Build history of the part. All positions in model axes, mm. A direction names the side the tool comes from. Coordinates: 2 decimals unless noted, no trailing zeros. Order: outer loops, then holes, each group sorted by start corner. A loop starts at its lowest first (then second) coordinate and runs counter-clockwise, first axis right, second up. Notation, with made-up numbers: M 41,-20 L 68,-20 A28 ccw 68,16 Z; hole C 10.5,-1 d6. An arc over 180 degrees is marked long. Write item = value, one per line. Start each with the question number.
Q1. Drill centre lines: probe 1 along X at (y, z) = (0.95, 6.17); probe 2 along Z at (x, y) = (5, 0.1); probe 3 along Z at (x, y) = (4.5, 0.5). Where is each one in solid material? Low to high.
Q2. Band-saw the part on D-D on x = 6.5. Write the cut outline in (y, z).
Q3. Band-saw the part on B-B on z = 4. Write the cut outline in (x, y), plus the area to 3 significant figures.
Q4. 3-axis set-ups, long thin cutter, end or side, ignore diameter. For faces 5 (the face through (15.51, 1.08, 3.37)), 6 (the face through (4, 1, 12.65)): which of +Z, -Z, +X, -X, +Y, -Y reach the whole face in a straight line?
Q5. Pull direction Z, two halves, no side cores. Call faces 1 (the face through (3.51, 1.08, 3.37)), 2 (the face through (20, 1, 17)), 3 (the face through (9.85, 1.08, 27)), 4 (the face through (10, 1, 0)): released by +Z, released by -Z, zero draft, split by the parting line, or undercut.
Q6. Band-saw the part on C-C on y = 1.65. Write the cut outline in (x, z).
Q7. Pin check, flat tip, straight feed: P1, Ø1.4, axis at x = 4, z = 4, coming from the -Y side. Stop position of the tip, or through.
Q8. Band-saw the part on A-A on x = 4. Write the cut outline in (y, z).
```python
from build123d import *

# Parameters (mm, degrees)
SKETCH_1_R      = 0.8
SKETCH_1_R_2    = 0.4
EXTRUDE_1_DEPTH = 2.2


with BuildPart() as part:
    # 草图1 → 凸台-拉伸1 (new body)
    with BuildSketch(Plane(origin=(0, 0, 0), x_dir=(1, 0, 0), z_dir=(0, 1, 0))):
        with BuildLine():
            Line((20, 0), (0, 0))
            Line((0, 0), (0, -12.65))
            Line((0, -12.65), (8.608058909, -12.65))
            ThreePointArc((8.608058909, -12.65), (12.283882181, -13.116117819), (14, -16.4))
            ThreePointArc((14, -16.4), (12.283882181, -19.683882181), (8.608058909, -20.15))
            Line((8.608058909, -20.15), (0, -20.15))
            Line((0, -20.15), (0, -32.8))
            Line((0, -32.8), (20, -32.8))
            Line((20, -32.8), (20, 0))
        make_face()
        with Locations(Location((4, -28.8, 0), (0, 0, 270))):
            Circle(SKETCH_1_R, mode=Mode.SUBTRACT)
        with Locations(Location((10, -26.63, 0), (0, 0, 270))):
            Circle(SKETCH_1_R_2, mode=Mode.SUBTRACT)
        with Locations(Location((16, -28.8, 0), (0, 0, 270))):
            Circle(SKETCH_1_R, mode=Mode.SUBTRACT)
        with Locations(Location((4, -4, 0), (0, 0, 270))):
            Circle(SKETCH_1_R, mode=Mode.SUBTRACT)
        with Locations(Location((10, -6.17, 0), (0, 0, 270))):
            Circle(SKETCH_1_R_2, mode=Mode.SUBTRACT)
        with Locations(Location((16, -4, 0), (0, 0, 270))):
            Circle(SKETCH_1_R, mode=Mode.SUBTRACT)
    extrude(amount=EXTRUDE_1_DEPTH)


solid = part.part
```
Recorded:
q1.probe_1 = 0 to 9.6, 10.4 to 20
q1.probe_2 = 0 to 12.65, 20.15 to 32.8
q1.probe_3 = 0 to 3.38, 4.62 to 12.65, 20.15 to 28.18, 29.42 to 32.8
q2.outline = M 0,0 L 2.2,0 L 2.2,12.65 L 0,12.65 Z; M 0,20.15 L 2.2,20.15 L 2.2,32.8 L 0,32.8 Z
q3.outline = M 0,0 L 3.2,0 L 3.2,2.2 L 0,2.2 Z; M 4.8,0 L 15.2,0 L 15.2,2.2 L 4.8,2.2 Z; M 16.8,0 L 20,0 L 20,2.2 L 16.8,2.2 Z
q3.area = 37.0 mm2
q4.face_5 = +Y, -Y
q4.face_6 = -X, +Y, -Y
q5.face_1 = undercut
q5.face_2 = zero draft
q5.face_3 = undercut
q5.face_4 = released by -Z
q6.outline = M 0,0 L 20,0 L 20,32.8 L 0,32.8 L 0,20.15 L 8.61,20.15 A4 cw long 8.61,12.65 L 0,12.65 Z; hole C 4,4 d1.6; hole C 4,28.8 d1.6; hole C 10,6.17 d0.8; hole C 10,26.63 d0.8; hole C 16,4 d1.6; hole C 16,28.8 d1.6
q7.P1 = through
q8.outline = M 0,0 L 2.2,0 L 2.2,3.2 L 0,3.2 Z; M 0,4.8 L 2.2,4.8 L 2.2,12.65 L 0,12.65 Z; M 0,20.15 L 2.2,20.15 L 2.2,28 L 0,28 Z; M 0,29.6 L 2.2,29.6 L 2.2,32.8 L 0,32.8 Z
